Could you check a few things on this model? Use its own coordinates, in mm. Face numbers are marked on the shaded views. A direction names the side the tool comes from. Coordinates: 2 decimals unless noted, no trailing zeros. Write each loop counter-clockwise with the first axis right and the second up, starting at its lowest first coordinate (ties: lowest second). Pieces come first, ordered by that corner, then holes.
Item 1: I want a section at C-C on y = 17.5. Please give me the cut outline in (x, z).
Item 2: I want a section at B-B on x = 21.5. Please give me the cut outline in (y, z), then the cut area to 3 significant figures.
Item 3: Thinking about a two-plate mould opening in Y: for the marked faces 3, 4 and 5, which applies, +Y half, -Y half, draft (parallel to the pull), parting line (faces both ways), or undercut?
Item 4: I want a section at A-A on z = -57. Please give me the cut outline in (x, y).
Item 5: For P1, Ø8, axis at x = 39, y = -38, coming from the -Z side, with a flat end and sliding along its axis, tell me the tip position at first contact or that it passes through.
Item 6: Which directions (+Z, -Z, +X, -X, +Y, -Y) give clear straight access to the entire face, cutting with the end or side of a thin tool? Please do the marked faces 1 and 2.
Item 7: If I drill on probe 1 along Y at (x, z) = (6, -49); probe 2 along X at (y, z) = (-44.5, -47.5); probe 3 along Z at (x, y) = (48, 31), over which ranges is the centre line in solid material (lowest first)?
from build123d import *

# Parameters (mm, degrees)
F0_W     = 120.4
F0_H     = 101.6
F1_DEPTH = 119.75
F2_T     = -2.54
F3_R     = 5.08


with BuildPart() as f1:
    # F0 (on Top) → F1 (new body)
    with BuildSketch(Plane.XY):
        with Locations((1.22794, -2.425997)):
            Rectangle(F0_W, F0_H)
    extrude(amount=-F1_DEPTH)

    # F2
    f2_openings = [f1.faces().sort_by_distance(p)[0] for p in [
        (1.22794, -2.425997, -119.75),
    ]]
    offset(amount=F2_T, openings=f2_openings)

    # F3
    f3_edges = [f1.edges().sort_by_distance(p)[0] for p in [
        (61.42794, 48.374003, -59.875),
        (-58.97206, 48.374003, -59.875),
        (-58.97206, -53.225997, -59.875),
        (61.42794, -53.225997, -59.875),
    ]]
    fillet(f3_edges, radius=F3_R)


solid = f1.part
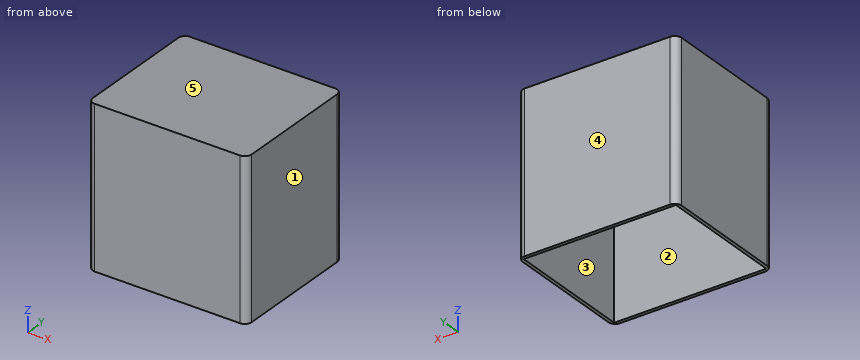
Response values:
1. outline: (-58.97, -119.75) - (-56.43, -119.75) - (-56.43, -2.54) - (58.89, -2.54) - (58.89, -119.75) - (61.43, -119.75) - (61.43, 0) - (-58.97, 0) - close
2. outline: (-53.23, -119.75) - (-50.69, -119.75) - (-50.69, -2.54) - (45.83, -2.54) - (45.83, -119.75) - (48.37, -119.75) - (48.37, 0) - (-53.23, 0) - close
2. area: 853 mm2
3. face 3: undercut
3. face 4: +Y half
3. face 5: draft
4. outline: (-58.97, -48.15) arc R5.08 ccw to (-53.89, -53.23) - (56.35, -53.23) arc R5.08 ccw to (61.43, -48.15) - (61.43, 43.29) arc R5.08 ccw to (56.35, 48.37) - (-53.89, 48.37) arc R5.08 ccw to (-58.97, 43.29) - close; hole (-56.43, -50.69) - (58.89, -50.69) - (58.89, 45.83) - (-56.43, 45.83) - close
5. P1: stops at z = -2.54
6. face 1: +Z, -Z, +X, +Y, -Y
6. face 2: -Z
7. probe 1: y = -53.23 to -50.69, 45.83 to 48.37
7. probe 2: x = -58.97 to -56.43, 58.89 to 61.43
7. probe 3: z = -2.54 to 0
